Read the model definition and answer for the solid it produces. Units are mm, in the model's axes. A direction names the side the tool comes from. Coordinates: 2 decimals unless noted, no trailing zeros. Write each loop counter-clockwise with the first axis right and the second up, starting at its lowest first coordinate (ties: lowest second). Pieces come first, ordered by that corner, then holes. Notation, with made-up numbers: (-18, 32.5) - (38, 32.5) arc R24 ccw to (38, 55.5) - close; hole circle Ø8 at (83, -12.75). An arc over 180 degrees is marked (long way). Return JSON: item names as keys, results as strings.
```python
from build123d import *

# Parameters (mm, degrees)
SKETCH1_R                = 13.75
SKETCH1_R_2              = 4.15
BOSS_EXTRUDE1_DEPTH      = 2.5
SKETCH2_R                = 6.5
SKETCH2_R_2              = 4.15
BOSS_EXTRUDE2_DEPTH      = 2.5
CUT_EXTRUDE1_DEPTH       = 21.077973005
FILLET1_R                = 0.5
CIRPATTERN1_COUNT        = 16
FILLET1_OF_CIRPATTERN1_R = 0.5


with BuildPart() as part:
    # Sketch1 → Boss-Extrude1 (new body)
    with BuildSketch(Plane.XY):
        Circle(SKETCH1_R)
        Circle(SKETCH1_R_2, mode=Mode.SUBTRACT)
    extrude(amount=BOSS_EXTRUDE1_DEPTH)

    # Sketch2 → Boss-Extrude2 (add)
    with BuildSketch(Plane.XY.offset(2.5)):
        Circle(SKETCH2_R)
        Circle(SKETCH2_R_2, mode=Mode.SUBTRACT)
    extrude(amount=BOSS_EXTRUDE2_DEPTH)

    # Sketch5 → Cut-Extrude1 (cut, through all)
    with BuildSketch(Plane.XY):
        with BuildLine():
            Line((0, 12.75), (0, 7.5))
            ThreePointArc((0, 7.5), (0.735128552, 7.46388545), (1.463177415, 7.355889603))
            Line((1.463177415, 7.355889603), (2.487401606, 12.505012325))
            ThreePointArc((2.487401606, 12.505012325), (1.249718539, 12.688605265), (0, 12.75))
        make_face()
    cut_extrude1 = extrude(amount=CUT_EXTRUDE1_DEPTH, mode=Mode.SUBTRACT)

    # Fillet1
    fillet1_edges = [part.edges().sort_by_distance(p)[0] for p in [
        (0, 7.5, 1.25),
        (1.463177415, 7.355889603, 1.25),
        (2.487401606, 12.505012325, 1.25),
        (0, 12.75, 1.25),
    ]]
    fillet(fillet1_edges, radius=FILLET1_R)

    # CirPattern1: Cut-Extrude1 ×16 about axis
    cirpattern1_axis = Axis((0, 0, 0), (0, 0, 1))
    for i in range(1, CIRPATTERN1_COUNT):
        add(cut_extrude1.rotate(cirpattern1_axis, i * 360 / CIRPATTERN1_COUNT), mode=Mode.SUBTRACT)

    # Fillet1 of CirPattern1
    fillet1_of_cirpattern1_edges = [part.edges().sort_by_distance(p)[0] for p in [
        (-2.870125743, 6.929096494, 1.25),
        (-1.463177415, 7.355889603, 1.25),
        (-2.487401606, 12.505012325, 1.25),
        (-4.879213763, 11.77946404, 1.25),
        (-5.303300859, 5.303300859, 1.25),
        (-4.166776748, 6.236022092, 1.25),
        (-7.083520471, 10.601237557, 1.25),
        (-9.01561146, 9.01561146, 1.25),
        (-6.929096494, 2.870125743, 1.25),
        (-6.236022092, 4.166776748, 1.25),
        (-10.601237557, 7.083520471, 1.25),
        (-11.77946404, 4.879213763, 1.25),
        (-7.5, 0, 1.25),
        (-7.355889603, 1.463177415, 1.25),
        (-12.505012325, 2.487401606, 1.25),
        (-12.75, 0, 1.25),
        (-6.929096494, -2.870125743, 1.25),
        (-7.355889603, -1.463177415, 1.25),
        (-12.505012325, -2.487401606, 1.25),
        (-11.77946404, -4.879213763, 1.25),
        (-5.303300859, -5.303300859, 1.25),
        (-6.236022092, -4.166776748, 1.25),
        (-10.601237557, -7.083520471, 1.25),
        (-9.01561146, -9.01561146, 1.25),
        (-2.870125743, -6.929096494, 1.25),
        (-4.166776748, -6.236022092, 1.25),
        (-7.083520471, -10.601237557, 1.25),
        (-4.879213763, -11.77946404, 1.25),
        (0, -7.5, 1.25),
        (-1.463177415, -7.355889603, 1.25),
        (-2.487401606, -12.505012325, 1.25),
        (0, -12.75, 1.25),
        (2.870125743, -6.929096494, 1.25),
        (1.463177415, -7.355889603, 1.25),
        (2.487401606, -12.505012325, 1.25),
        (4.879213763, -11.77946404, 1.25),
        (5.303300859, -5.303300859, 1.25),
        (4.166776748, -6.236022092, 1.25),
        (7.083520471, -10.601237557, 1.25),
        (9.01561146, -9.01561146, 1.25),
        (6.929096494, -2.870125743, 1.25),
        (6.236022092, -4.166776748, 1.25),
        (10.601237557, -7.083520471, 1.25),
        (11.77946404, -4.879213763, 1.25),
        (7.5, 0, 1.25),
        (7.355889603, -1.463177415, 1.25),
        (12.505012325, -2.487401606, 1.25),
        (12.75, 0, 1.25),
        (6.929096494, 2.870125743, 1.25),
        (7.355889603, 1.463177415, 1.25),
        (12.505012325, 2.487401606, 1.25),
        (11.77946404, 4.879213763, 1.25),
        (5.303300859, 5.303300859, 1.25),
        (6.236022092, 4.166776748, 1.25),
        (10.601237557, 7.083520471, 1.25),
        (9.01561146, 9.01561146, 1.25),
        (2.870125743, 6.929096494, 1.25),
        (4.166776748, 6.236022092, 1.25),
        (7.083520471, 10.601237557, 1.25),
        (4.879213763, 11.77946404, 1.25),
    ]]
    fillet(fillet1_of_cirpattern1_edges, radius=FILLET1_OF_CIRPATTERN1_R)


solid = part.part
```
(1) Which of the six approach directions +Z, -Z, +X, -X, +Y, -Y give full straight-line access (tool end or side, diameter ignored) to faces 1 (the face through (6, -3, 2.5)), 2 (the face through (9.37, -3.88, 1.23))?
Answer:
{"face 1": "+Z", "face 2": "+Z, -Z"}
(2) A cutting plane is placed at A-A (z = 0.5). State how many separate pieces and enclosed holes the cut face has, and give its area (3 significant figures).
Answer:
{"separate pieces": "1", "enclosed holes": "17", "area": "376 mm²"}
(3) Straight lines are drawn through the part: line 1 (Y direction, x = 0, z = 3); line 2 (Y direction, x = -1, z = 2.4); line 3 (X direction, y = 3.75, z = 1.6). For each, find the intervals that lie inside material, in ascending order. Write a range as from..to.
Answer:
{"line 1": "-6.5..-4.15, 4.15..6.5", "line 2": "-13.71..-12.71, -7.43..-4.03, 4.03..13.71", "line 3": "-13.23..-9.05, -6.5..-1.78, 1.78..9.05, 12.19..13.23"}
(4) A cutting plane is placed at B-B (z = 3.6). Determine the outline of the cut face in (x, y), and give its area (3 significant figures).
Answer:
{"outline": "circle Ø13 at (0, 0); hole circle Ø8.3 at (0, 0)", "area": "78.6 mm²"}
(5) Determine the mould class of faces 3 (the face through (-2.981, -13.423, 1.232)), 4 (the face through (10, 0, 1)), 5 (the face through (-3.88, 9.37, 1.23)), 6 (the face through (2.9, 3.2, 0)) for opening direction Y: +Y half, -Y half, draft (parallel to the pull), parting line (faces both ways), or undercut.
Answer:
{"face 3": "parting line", "face 4": "undercut", "face 5": "undercut", "face 6": "draft"}
(6) Flat-ended cylindrical pins translate along their axes: P1, Ø0.8, axis at x = 9.5, z = 1.5, coming from the -Y side; P2, Ø3, axis at y = -10.5, z = 1.5, coming from the -X side; P3, Ø5, axis at x = -3.5, y = 10.5, coming from the +Z side. Find the tip coordinate at first contact, or state that the pin passes through.
Answer:
{"P1": "y = -10.31", "P2": "x = -10.4", "P3": "z = 2.5"}
